CAD build for the part. Positions are in the model's coordinates, mm. Coordinates: 2 decimals unless noted, no trailing zeros. Loops run counter-clockwise (first coordinate to the right, second up) from the corner with the lowest first, then second, coordinate; pieces in that order, holes last. Notation, with made-up numbers: (47, 53) -> (92, 53) arc R15 ccw to (92, 70) -> close; hole circle Ø7 at (71, 40.25). An arc over 180 degrees is marked (long way). Write each question's results on one line, items separated by ' | '.
from build123d import *

# Parameters (mm, degrees)
BOSS_EXTRUDE1_DEPTH   = 4.7625
SKETCH2_R             = 2.2225
CUT_EXTRUDE1_DEPTH    = 73.495756083
SKETCH3_R             = 2.2225
CUT_EXTRUDE2_DEPTH    = 73.495756083
CIRPATTERN1_START     = -4.7625
CIRPATTERN1_OUTLINE_R = 2.2225
CIRPATTERN1_DEPTH     = 9.525
CIRPATTERN2_START     = -4.7625
CIRPATTERN2_OUTLINE_R = 2.2225
CIRPATTERN2_DEPTH     = 9.525
BOSS_EXTRUDE2_DEPTH   = 9.525
FILLET1_R             = 6.35
FILLET2_R             = 25.4


# Read off the part's stored shape, not the designer's step: CirPattern1, CirPattern2
with BuildPart() as part:
    # Sketch1 → Boss-Extrude1 (new, symmetric)
    with BuildSketch(Plane(origin=(0, 0, 0), x_dir=(1, 0, 0), z_dir=(0, 1, 0))):
        with BuildLine():
            Line((-44.760744171, 30.1625), (55.879098004, 30.1625))
            ThreePointArc((55.879098004, 30.1625), (63.467858945, -2.02011904), (53.847850236, -33.655))
            Line((53.847850236, -33.655), (29.036932948, -33.655))
            Line((29.036932948, -33.655), (-36.477972806, -25.4))
            Line((-36.477972806, -25.4), (-47.625, -25.4))
            ThreePointArc((-47.625, -25.4), (-53.903425523, 2.778730272), (-44.760744171, 30.1625))
        make_face()
    extrude(amount=BOSS_EXTRUDE1_DEPTH, both=True)

    # Sketch2 → Cut-Extrude1 (cut, through all)
    with BuildSketch(Plane(origin=(0, 4.7625, 0), x_dir=(1, 0, 0), z_dir=(0, 1, 0))):
        with Locations(Location((-49.2125, 0, 0), (0, 0, 270))):
            Circle(SKETCH2_R)
    extrude(amount=-CUT_EXTRUDE1_DEPTH, mode=Mode.SUBTRACT)

    # Sketch3 → Cut-Extrude2 (cut, through all)
    with BuildSketch(Plane(origin=(0, 4.7625, 0), x_dir=(1, 0, 0), z_dir=(0, 1, 0))):
        with Locations(Location((53.975, 0, 0), (0, 0, 270))):
            Circle(SKETCH3_R)
    extrude(amount=-CUT_EXTRUDE2_DEPTH, mode=Mode.SUBTRACT)

    # CirPattern1 outline → CirPattern1 (cut)
    with BuildSketch(Plane(origin=(0, 0, 0), x_dir=(1, 0, 0), z_dir=(0, 1, 0)).offset(CIRPATTERN1_START)):
        with Locations((-47.750678429, 11.905581287)):
            Circle(CIRPATTERN1_OUTLINE_R)
        with Locations((-43.452058414, 23.103869284)):
            Circle(CIRPATTERN1_OUTLINE_R)
        with Locations((-48.137088801, -10.231854084)):
            Circle(CIRPATTERN1_OUTLINE_R)
        with Locations((-44.957855834, -20.016527047)):
            Circle(CIRPATTERN1_OUTLINE_R)
    extrude(amount=CIRPATTERN1_DEPTH, mode=Mode.SUBTRACT)

    # CirPattern2 outline → CirPattern2 (cut)
    with BuildSketch(Plane(origin=(0, 0, 0), x_dir=(1, 0, 0), z_dir=(0, 1, 0)).offset(CIRPATTERN2_START)):
        with Locations((52.591624247, 12.141733158)):
            Circle(CIRPATTERN2_OUTLINE_R)
        with Locations((48.512408649, 23.661082648)):
            Circle(CIRPATTERN2_OUTLINE_R)
        with Locations((52.135846474, -13.969757959)):
            Circle(CIRPATTERN2_OUTLINE_R)
        with Locations((46.743721169, -26.9875)):
            Circle(CIRPATTERN2_OUTLINE_R)
    extrude(amount=CIRPATTERN2_DEPTH, mode=Mode.SUBTRACT)

    # Sketch4 → Boss-Extrude2 (add, through all)
    with BuildSketch(Plane(origin=(0, 4.7625, 0), x_dir=(1, 0, 0), z_dir=(0, 1, 0))):
        with BuildLine():
            Line((-48.917962805, -22.810820677), (-73.619827915, 30.1625))
            Line((-73.619827915, 30.1625), (-44.760744171, 30.1625))
            ThreePointArc((-44.760744171, 30.1625), (-53.809555017, 4.222844291), (-48.917962805, -22.810820677))
        make_face()
    extrude(amount=-BOSS_EXTRUDE2_DEPTH)

    # Fillet1
    fillet1_edges = [part.edges().sort_by_distance(p)[0] for p in [
        (55.879098004, 0, -30.1625),
        (53.847850236, 0, 33.655),
        (-47.625, 0, 25.4),
        (-73.619827915, 0, -30.1625),
    ]]
    fillet(fillet1_edges, radius=FILLET1_R)

    # Fillet2
    fillet2_edges = [part.edges().sort_by_distance(p)[0] for p in [
        (29.036932948, 0, 33.655),
        (-36.477972806, 0, 25.4),
    ]]
    fillet(fillet2_edges, radius=FILLET2_R)


solid = part.part
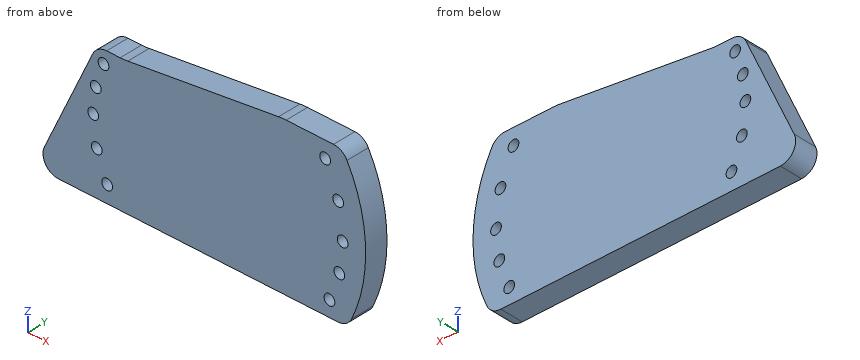
1) Pin check, flat tips, straight feed: pin 1 (3.5 mm diameter, centred on x = -48.14, z = 10.23, fed in from -Y); pin 2 (1 mm diameter, centred on y = 0, z = 8.5, fed in from +X); pin 3 (5 mm diameter, centred on x = -44.96, z = 20.02, fed in from +Y); pin 4 (2 mm diameter, centred on y = 2.5, z = -13.5, fed in from +X). Stop position of each tip, or through.
Outcome:
pin 1: passes through | pin 2: stops at x = 62.99 | pin 3: stops at y = 4.76 | pin 4: stops at x = 62.26
2) Slice it at D-D (z = -16). Write the cut outline in (x, y).
Outcome:
outline: (-67.02, -4.76) -> (61.45, -4.76) -> (61.45, 4.76) -> (-67.02, 4.76) -> close
3) Slice it at B-B (y = -0.5). Count the separate pieces of the cut face and the enclosed holes in it, then the cut area to 3 significant figures.
Outcome:
separate pieces: 1 | enclosed holes: 10 | area: 7,090 mm^2
4) Drill centre lines: L1, parallel to X at y = 4.5, z = -12; L2, parallel to Z at x = -49.5, y = 1; L3, parallel to X at y = -3.5, z = -22. Where is each one in solid material? Low to high. Write a range as from..to.
Outcome:
L1: x = -65.15..-49.97, -45.53..50.37, 54.81..62.36 | L2: z = -30.16..-13.28, -10.53..-2.2, 2.2..8.48, 11.99..21.56 | L3: x = -69.74..-45.38, -41.52..47.04, 49.99..59.57
5) Slice it at A-A (z = 0). Write the cut outline in (x, y) (1 decimal).
Outcome:
outline: (-59.6, -4.8) -> (-51.4, -4.8) -> (-51.4, 4.8) -> (-59.6, 4.8) -> close; (-47, -4.8) -> (51.8, -4.8) -> (51.8, 4.8) -> (-47, 4.8) -> close; (56.2, -4.8) -> (63.5, -4.8) -> (63.5, 4.8) -> (56.2, 4.8) -> close
6) Slice it at C-C (x = -57.5). Write the cut outline in (y, z).
Outcome:
outline: (-4.76, -30.16) -> (4.76, -30.16) -> (4.76, 4.41) -> (-4.76, 4.41) -> close
